Here's how the part is built. I have some questions about the finished solid (model axes, mm). Face numbers are marked on the shaded views. A direction names the side the tool comes from. Coordinates: 2 decimals unless noted, no trailing zeros. Write each loop counter-clockwise with the first axis right and the second up, starting at its lowest first coordinate (ties: lowest second). Pieces come first, ordered by that corner, then holes.
```python
from build123d import *

# Parameters (mm, degrees)
SKETCH1_W           = 31.75
SKETCH1_H           = 31.75
BOSS_EXTRUDE1_DEPTH = 17.145
SKETCH2_R           = 4.445
CUT_EXTRUDE1_DEPTH  = 49.063250254
SKETCH3_W           = 26.416
SKETCH3_H           = 6.35
CUT_EXTRUDE2_DEPTH  = 49.063250254
SKETCH4_W           = 28.575
SKETCH4_H           = 9.398
CUT_EXTRUDE3_DEPTH  = 49.063250254
FILLET2_DEPTH       = 31.75
FILLET2_2_DEPTH     = 2.667
FILLET2_START       = 29.083
FILLET2_3_DEPTH     = 2.667


with BuildPart() as part:
    # Sketch1 → Boss-Extrude1 (new body)
    with BuildSketch(Plane(origin=(0, 0, 0), x_dir=(1, 0, 0), z_dir=(0, 1, 0))):
        with Locations((15.875, 15.875)):
            Rectangle(SKETCH1_W, SKETCH1_H)
    extrude(amount=BOSS_EXTRUDE1_DEPTH)

    # Sketch2 → Cut-Extrude1 (cut, through all)
    with BuildSketch(Plane(origin=(0, 17.145, 0), x_dir=(1, 0, 0), z_dir=(0, 1, 0))):
        with Locations(Location((15.875, 15.875, 0), (0, 0, 270))):
            Circle(SKETCH2_R)
    extrude(amount=-CUT_EXTRUDE1_DEPTH, mode=Mode.SUBTRACT)

    # Sketch3 → Cut-Extrude2 (cut, through all)
    with BuildSketch(Plane.XY):
        with Locations((15.875, 3.175)):
            Rectangle(SKETCH3_W, SKETCH3_H)
    extrude(amount=-CUT_EXTRUDE2_DEPTH, mode=Mode.SUBTRACT)

    # Sketch4 → Cut-Extrude3 (cut, through all)
    with BuildSketch(Plane.ZY):
        with Locations((-15.875, 10.8585)):
            Rectangle(SKETCH4_W, SKETCH4_H)
    extrude(amount=-CUT_EXTRUDE3_DEPTH, mode=Mode.SUBTRACT)

    # Fillet2: read off the stored shape, not the designer's step
    # Fillet2 outline → Fillet2 (add)
    with BuildSketch(Plane.YZ):
        with BuildLine():
            Line((6.35, -26.7335), (6.35, -30.1625))
            Line((6.35, -30.1625), (15.5575, -30.1625))
            Line((15.5575, -30.1625), (15.5575, -25.4))
            ThreePointArc((15.5575, -25.4), (14.184972345, -28.745070067), (10.8585, -30.162076648))
            ThreePointArc((10.8585, -30.162076648), (8.039162939, -29.190864906), (6.35, -26.7335))
        make_face()
        with BuildLine():
            ThreePointArc((10.8585, -1.587923352), (14.184972345, -3.004929933), (15.5575, -6.35))
            Line((15.5575, -6.35), (15.5575, -1.5875))
            Line((15.5575, -1.5875), (6.35, -1.5875))
            Line((6.35, -1.5875), (6.35, -5.0165))
            ThreePointArc((6.35, -5.0165), (8.039162939, -2.559135094), (10.8585, -1.587923352))
        make_face()
    extrude(amount=FILLET2_DEPTH)

    # Fillet2 2 outline → Fillet2 2 (add)
    with BuildSketch(Plane.YZ):
        with BuildLine():
            Line((6.1595, -30.1625), (6.35, -30.1625))
            Line((6.35, -30.1625), (6.35, -26.7335))
            ThreePointArc((6.35, -26.7335), (6.207365536, -26.073519209), (6.1595, -25.4))
            Line((6.1595, -25.4), (6.1595, -30.1625))
        make_face()
        with BuildLine():
            Line((6.1595, -1.5875), (6.1595, -6.35))
            ThreePointArc((6.1595, -6.35), (6.207365536, -5.676480791), (6.35, -5.0165))
            Line((6.35, -5.0165), (6.35, -1.5875))
            Line((6.35, -1.5875), (6.1595, -1.5875))
        make_face()
    extrude(amount=FILLET2_2_DEPTH)

    # Fillet2 3 outline → Fillet2 3 (add)
    with BuildSketch(Plane.YZ.offset(FILLET2_START)):
        with BuildLine():
            Line((6.1595, -30.1625), (6.35, -30.1625))
            Line((6.35, -30.1625), (6.35, -26.7335))
            ThreePointArc((6.35, -26.7335), (6.207365536, -26.073519209), (6.1595, -25.4))
            Line((6.1595, -25.4), (6.1595, -30.1625))
        make_face()
        with BuildLine():
            Line((6.1595, -1.5875), (6.1595, -6.35))
            ThreePointArc((6.1595, -6.35), (6.207365536, -5.676480791), (6.35, -5.0165))
            Line((6.35, -5.0165), (6.35, -1.5875))
            Line((6.35, -1.5875), (6.1595, -1.5875))
        make_face()
    extrude(amount=FILLET2_3_DEPTH)


solid = part.part
```
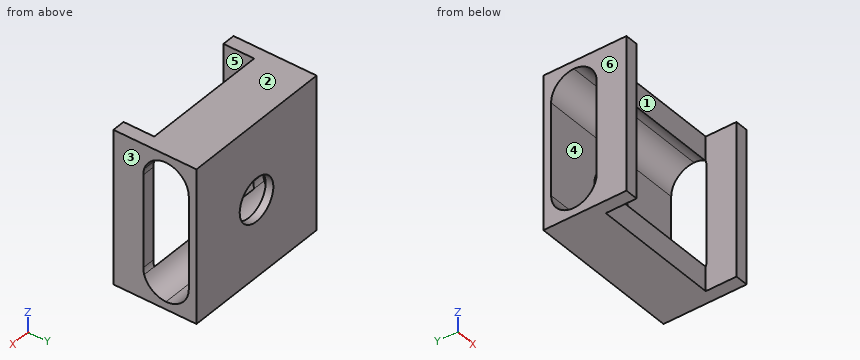
1) We'd pull the mould along X, two halves only. Please class the marked faces 1, 2 and 3: pulls with the +X half, pulls with the -X half, needs draft (parallel to the pull), parting line crosses it, or undercut.
Values follow:
face 1: undercut
face 2: needs draft
face 3: pulls with the +X half
2) I need wall thicknesses on probe 1 along Y at (x, z) = (29.5, -21.5) (1 decimal); probe 2 along X at (y, z) = (4, -10.5); probe 3 along Z at (x, y) = (4, 11). Which ranges of each line are inside material? Lowest first, please.
Values follow:
probe 1: y = 0 to 6.2, 15.6 to 17.1
probe 2: x = 0 to 2.67, 29.08 to 31.75
probe 3: z = -31.75 to -30.16, -1.59 to 0
3) Imagine slicing it at B-B on y = 1.75. Please give me the cut outline in (x, z).
Values follow:
outline: (0, -31.75) - (2.67, -31.75) - (2.67, 0) - (0, 0) - close; (29.08, -31.75) - (31.75, -31.75) - (31.75, 0) - (29.08, 0) - close
4) Will these pins go through, and if not, where does the flat tip stop? pin 1 (4 mm diameter, centred on x = 13.5, z = -26, fed in from -Y); pin 2 (14 mm diameter, centred on x = 15.875, z = -15.875, fed in from -Y); pin 3 (7 mm diameter, centred on y = 2, z = -11, fed in from -X).
Values follow:
pin 1: stops at y = 6.35
pin 2: stops at y = 15.56
pin 3: stops at x = 0
5) On a 3-axis mill with a long thin cutter (end or side, diameter ignored), from which of +Z, -Z, +X, -X, +Y, -Y can I reach the whole of each face in a straight line? I mean the marked faces 4, 5 and 6. Say none if no direction works.
Values follow:
face 4: +X, -X
face 5: +Z, -Z, -Y
face 6: +Z, -Z, -X, +Y, -Y
6) Imagine slicing it at C-C on z = -24. Count the separate pieces of the cut face and the enclosed holes in it, then the cut area to 3 significant figures.
Values follow:
separate pieces: 3
enclosed holes: 0
area: 83.3 mm2
